```python
from build123d import *

# Parameters (mm, degrees)
SKETCH1_W           = 75
SKETCH1_H           = 17
BOSS_EXTRUDE1_DEPTH = 1.5
SKETCH2_W           = 4
SKETCH2_H           = 17
SKETCH2_W_2         = 1.969333236
BOSS_EXTRUDE2_DEPTH = 5.3
SKETCH3_W           = 14.056018955
SKETCH3_H           = 1.3
CUT_EXTRUDE1_DEPTH  = 2.1
SKETCH4_W           = 1.969333236
SKETCH4_H           = 17
BOSS_EXTRUDE3_DEPTH = 3
SKETCH5_W           = 7.906104095
SKETCH5_H           = 3.4
CUT_EXTRUDE3_DEPTH  = 33


with BuildPart() as part:
    # Sketch1 → Boss-Extrude1 (new body)
    with BuildSketch(Plane(origin=(0, 0, 0), x_dir=(1, 0, 0), z_dir=(0, 1, 0))):
        with Locations((-3.550742823, -7.98686986)):
            Rectangle(SKETCH1_W, SKETCH1_H)
    extrude(amount=BOSS_EXTRUDE1_DEPTH)

    # Sketch2 → Boss-Extrude2 (add)
    with BuildSketch(Plane(origin=(0, 1.5, 0), x_dir=(1, 0, 0), z_dir=(0, 1, 0))):
        with Locations((31.949257177, -7.98686986)):
            Rectangle(SKETCH2_W, SKETCH2_H)
        with Locations((-40.066076205, -7.98686986)):
            Rectangle(SKETCH2_W_2, SKETCH2_H)
    extrude(amount=BOSS_EXTRUDE2_DEPTH)

    # Sketch3 → Cut-Extrude1 (cut)
    with BuildSketch(Plane.ZY.offset(-29.949257177)):
        with Locations((8.014879338, 4.15)):
            Rectangle(SKETCH3_W, SKETCH3_H)
    extrude(amount=-CUT_EXTRUDE1_DEPTH, mode=Mode.SUBTRACT)

    # Sketch4 → Boss-Extrude3 (add)
    with BuildSketch(Plane(origin=(0, 6.8, 0), x_dir=(1, 0, 0), z_dir=(0, 1, 0))):
        with Locations((-40.066076205, -7.98686986)):
            Rectangle(SKETCH4_W, SKETCH4_H)
    extrude(amount=BOSS_EXTRUDE3_DEPTH)

    # Sketch5 → Cut-Extrude3 (cut)
    with BuildSketch(Plane(origin=(-39.081409587, 0, 0), x_dir=(0, 0, -1), z_dir=(1, 0, 0))):
        with Locations((-8.033817813, 6.7)):
            Rectangle(SKETCH5_W, SKETCH5_H)
    extrude(amount=-CUT_EXTRUDE3_DEPTH, mode=Mode.SUBTRACT)


solid = part.part
```
Geometry: final body of the model. Coordinates: model frame, mm. A direction names the side the tool comes from. Give positions to 0.01 mm unless a question says otherwise; leave off trailing zeros. Loops run counter-clockwise (first coordinate to the right, second up) from the corner with the lowest first, then second, coordinate; pieces in that order, holes last. Notation, with made-up numbers: (-10.75, 69) -> (-4.75, 69) arc R30 ccw to (-4.75, 98) -> close; hole circle Ø1 at (28, 18). An arc over 180 degrees is marked (long way). Return JSON: item names as keys, results as strings.
Item 1: Mould query, pull axis Y, two halves, no side actions, for faces 1 (the flat face through (-40, 7, 4.081)), 2 (the flat face through (-5, 1.5, 8)), 3 (the flat face through (33.949, 3, 8)). Classes: released by +Y, released by -Y, zero draft, split by the parting line, or undercut.
Filled in:
{"face 1": "undercut", "face 2": "released by +Y", "face 3": "zero draft"}
Item 2: Section A-A, the plane y = 2.75. Output: boundary loops of the cut face in (x, z), plus the area to 3 significant figures.
Filled in:
{"outline": "(-41.05, -0.51) -> (-39.08, -0.51) -> (-39.08, 16.49) -> (-41.05, 16.49) -> close; (29.95, -0.51) -> (33.95, -0.51) -> (33.95, 16.49) -> (29.95, 16.49) -> close", "area": "101 mm^2"}
Item 3: Section C-C, the plane y = 7.5. Output: boundary loops of the cut face in (x, z).
Filled in:
{"outline": "(-41.05, -0.51) -> (-39.08, -0.51) -> (-39.08, 4.08) -> (-41.05, 4.08) -> close; (-41.05, 11.99) -> (-39.08, 11.99) -> (-39.08, 16.49) -> (-41.05, 16.49) -> close"}
Item 4: Line query: line 1 (X direction, y = 3.75, z = 5.5); line 2 (Y direction, x = -33, z = 14.75); line 3 (X direction, y = 9.5, z = 8.5). Output: solid intervals per line, ascending.
Filled in:
{"line 1": "-41.05 to -39.08, 32.05 to 33.95", "line 2": "0 to 1.5", "line 3": "-41.05 to -39.08"}
Item 5: Access query for faces 4 (the flat face through (-7, 1, -0.513)), 5 (the flat face through (31, 3.5, 8)), 6 (the flat face through (-40, 8.4, 8)), 7 (the flat face through (29.949, 3, 8)), 8 (the flat face through (-40, 5, 8)). Directions: +Z, -Z, +X, -X, +Y, -Y. A direction counts if a zero-diameter tool reaches every point of the face in a straight line with its end or side. Return the directions, or none.
Filled in:
{"face 4": "-Z, +X, -X, +Y, -Y", "face 5": "none", "face 6": "+X, -X", "face 7": "+Z, -Z, +Y", "face 8": "-X"}
Item 6: Section D-D, the plane z = 14. Output: boundary loops of the cut face in (x, y), plus the area to 3 significant figures.
Filled in:
{"outline": "(-41.05, 0) -> (33.95, 0) -> (33.95, 6.8) -> (29.95, 6.8) -> (29.95, 4.8) -> (32.05, 4.8) -> (32.05, 3.5) -> (29.95, 3.5) -> (29.95, 1.5) -> (-39.08, 1.5) -> (-39.08, 9.8) -> (-41.05, 9.8) -> close", "area": "147 mm^2"}
Item 7: Pin query (flat end, axial travel): P1, Ø1.2, axis at x = 32, z = 7.5, coming from the +Y side; P2, Ø0.6, axis at x = -40.5, z = 9, coming from the -Y side; P3, Ø5, axis at x = -9, z = 7.5, coming from the +Y side. Return the tip coordinate at first contact, or that it passes through.
Filled in:
{"P1": "y = 6.8", "P2": "y = 0", "P3": "y = 1.5"}
Item 8: Section B-B, the plane z = 6.75. Output: boundary loops of the cut face in (x, y).
Filled in:
{"outline": "(-41.05, 0) -> (33.95, 0) -> (33.95, 6.8) -> (29.95, 6.8) -> (29.95, 4.8) -> (32.05, 4.8) -> (32.05, 3.5) -> (29.95, 3.5) -> (29.95, 1.5) -> (-39.08, 1.5) -> (-39.08, 5) -> (-41.05, 5) -> close; (-41.05, 8.4) -> (-39.08, 8.4) -> (-39.08, 9.8) -> (-41.05, 9.8) -> close"}
